```python
from build123d import *

# Parameters (mm, degrees)
F0_W          = 83.6295
F0_H          = 25.4
F2_R          = 2.38125
F2_R_2        = 3.2385
F2_R_3        = 6.35
F3_DEPTH      = 12.701
F3_DEPTH_BACK = 12.701
F4_W          = 25.4
F4_H          = 15.24


with BuildPart() as f1:
    # F0 (on Front) → F1 (revolve)
    with BuildSketch(Plane.XZ):
        with Locations((57.88025, 0)):
            Rectangle(F0_W, F0_H)
    revolve(axis=Axis((0, 0, 0), (0, 0, 1)))

    # F2 (on Top) → F3 (cut, two sides)
    with BuildSketch(Plane.XY) as f3_sk:
        with Locations((37.1475, 0)):
            Circle(F2_R)
        with Locations((-37.1475, 0)):
            Circle(F2_R_2)
        with Locations((0, 37.1475)):
            Circle(F2_R_3)
    extrude(amount=-F3_DEPTH, mode=Mode.SUBTRACT)
    extrude(f3_sk.sketch, amount=F3_DEPTH_BACK, mode=Mode.SUBTRACT)

    # F4 (on Front) → F5 (revolve, cut)
    with BuildSketch(Plane.XZ):
        with Locations((86.995, -5.08)):
            Rectangle(F4_W, F4_H)
    revolve(axis=Axis((0, 0, 0.5814679898), (0, 0, -1)), mode=Mode.SUBTRACT)


solid = f1.part
```
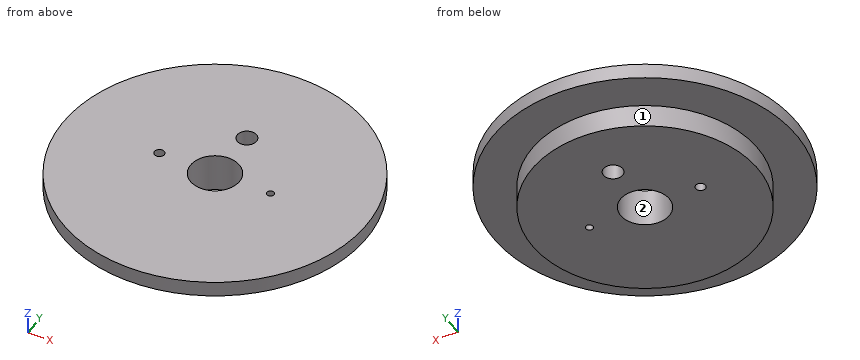
Part model, mm, in its own coordinate system. Face numbers are marked on the shaded views. A direction names the side the tool comes from. Coordinates: 2 decimals unless noted, no trailing zeros. Order: outer loops, then holes, each group sorted by start corner. A loop starts at its lowest first (then second) coordinate and runs counter-clockwise, first axis right, second up. Notation, with made-up numbers: (68, 27) -> (109, 27) arc R16 cw to (109, 36) -> close; hole circle Ø7 at (16, -21.5). An arc over 180 degrees is marked (long way). Put each result on its own line as item: value. Start each with the question number.
(1) Band-saw the part on A-A (x = 0). Give the cut face in (y, z) (1 decimal), then the cut area to 3 significant figures.
(2) Pin check, flat tips, straight feed: pin 1 Ø1.5 at (y, z) = (-58.5, -4.5) entering from -X; pin 2 Ø6 at (x, z) = (36.5, 6) entering from -Y; pin 3 Ø4 at (y, z) = (45.5, -6.5) entering from +X. Stop position of each tip, or through.
(3) Band-saw the part on B-B (y = 0). Give the cut face in (x, z) (1 decimal), then the cut area to 3 significant figures.
(4) Band-saw the part on C-C (z = 8.75). Count the separate pieces of the cut face and the enclosed holes in it, then the cut area to 3 significant figures.
(5) Band-saw the part on D-D (y = -23). Give the cut face in (x, z).
(6) Which spindle directions (+Z, -Z, +X, -X, +Y, -Y) get a long thin tool onto all of the face, cutting with end or side? Do the marked faces 1 and 2. Say none if no direction does.
(7) Probe line 1 along Y through (x, z) = (0, 6.75) (1 decimal); line 2 along Y through (x, z) = (0, -6.25) (1 decimal); line 3 along Z through (x, y) = (-89.5, 32.5). List the from-to ranges inside material, lowest first. Write a range as [from, to].
Determined:
1. outline: (-99.7, 2.5) -> (-74.3, 2.5) -> (-74.3, -12.7) -> (-16.1, -12.7) -> (-16.1, 12.7) -> (-99.7, 12.7) -> close; (16.1, -12.7) -> (30.8, -12.7) -> (30.8, 12.7) -> (16.1, 12.7) -> close; (43.5, -12.7) -> (74.3, -12.7) -> (74.3, 2.5) -> (99.7, 2.5) -> (99.7, 12.7) -> (43.5, 12.7) -> close
1. area: 3,150 mm²
2. pin 1: stops at x = -46.74
2. pin 2: stops at y = -93.9
2. pin 3: stops at x = 60.23
3. outline: (-99.7, 2.5) -> (-74.3, 2.5) -> (-74.3, -12.7) -> (-40.4, -12.7) -> (-40.4, 12.7) -> (-99.7, 12.7) -> close; (-33.9, -12.7) -> (-16.1, -12.7) -> (-16.1, 12.7) -> (-33.9, 12.7) -> close; (16.1, -12.7) -> (34.8, -12.7) -> (34.8, 12.7) -> (16.1, 12.7) -> close; (39.5, -12.7) -> (74.3, -12.7) -> (74.3, 2.5) -> (99.7, 2.5) -> (99.7, 12.7) -> (39.5, 12.7) -> close
3. area: 3,190 mm²
4. separate pieces: 1
4. enclosed holes: 4
4. area: 30,200 mm²
5. outline: (-97.01, 2.54) -> (-70.65, 2.54) -> (-70.65, -12.7) -> (70.65, -12.7) -> (70.65, 2.54) -> (97.01, 2.54) -> (97.01, 12.7) -> (-97.01, 12.7) -> close
6. face 1: -Z
6. face 2: +Z, -Z
7. line 1: y = [-99.7, -16.1], [16.1, 30.8], [43.5, 99.7]
7. line 2: y = [-74.3, -16.1], [16.1, 30.8], [43.5, 74.3]
7. line 3: z = [2.54, 12.7]
